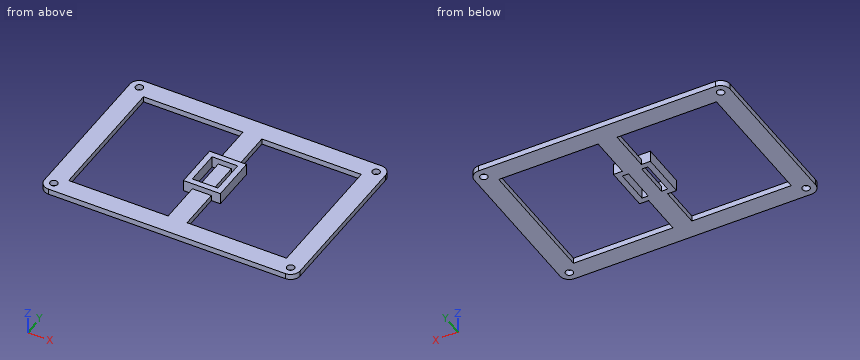
Autodesk Fusion 360 part; units mm, degrees
sketch "Boceto1" plane through (0, 0, 0) normal (0, 0, 1) x (1, 0, 0)
  line L0 (-6.75, 9.25) -> (6.75, 9.25)
  line L1 (6.75, 9.25) -> (6.75, -9.25)
  line L2 (6.75, -9.25) -> (-6.75, -9.25)
  line L3 (-6.75, -9.25) -> (-6.75, 9.25)
  line L4 (-6.75, 9.25) -> (6.75, -9.25) construction
  line L5 (6.75, 9.25) -> (-6.75, -9.25) construction
  line L6 (9.75, -12.25) -> (-9.75, -12.25)
  line L7 (-9.75, -12.25) -> (-9.75, 12.25)
  line L8 (-9.75, 12.25) -> (9.75, 12.25)
  line L9 (9.75, 12.25) -> (9.75, -12.25)
  line L10 (6.75, 0) -> (3.75, 0) construction
  line L11 (-6.75, 0) -> (-3.75, 0) construction
  line L12 (3.5, 0) -> (-3.5, 0)
  line L13 (-3.5, -9.25) -> (-3.5, 9.25)
  line L14 (3.5, -9.25) -> (3.5, 9.25)
  dimension "d1" = 13.5
  dimension "d2" = 18.5
  dimension "d3" = -3
  dimension "d4" = 3
  dimension "d5" = 3
  dimension "d6" = 7
extrude "Extruir1" add sketch "Boceto1" along normal blind 6
extrude "Extruir2" add sketch "Boceto1" along normal blind 3 contours L0 L12 L13 L14 | L2 L12 L13 L14
sketch "Boceto2" plane through (0, 0, 0) normal (0, 0, -1) x (1, 0, 0)
  line L0 (-3.5, -9.25) -> (-6.75, -9.25)
  line L1 (-6.75, -9.25) -> (-6.75, 9.25)
  line L2 (-6.75, 9.25) -> (-3.5, 9.25)
  line L3 (-3.5, 9.25) -> (-3.5, -9.25)
  line L4 (3.5, -9.25) -> (3.5, 9.25)
  line L5 (3.5, 9.25) -> (6.75, 9.25)
  line L6 (6.75, 9.25) -> (6.75, -9.25)
  line L7 (6.75, -9.25) -> (3.5, -9.25)
  line L8 (-9.75, -12.25) -> (9.75, -12.25)
  line L9 (9.75, -12.25) -> (9.75, 12.25)
  line L10 (9.75, 12.25) -> (-9.75, 12.25)
  line L11 (-9.75, 12.25) -> (-9.75, -12.25)
  line L12 (-67.5, 45) -> (67.5, 45)
  line L13 (67.5, 45) -> (67.5, -45)
  line L14 (67.5, -45) -> (-67.5, -45)
  line L15 (-67.5, -45) -> (-67.5, 45)
  line L16 (-67.5, 45) -> (67.5, -45) construction
  line L17 (67.5, 45) -> (-67.5, -45) construction
  line L18 (-67.5, 45) -> (-62.5, 45)
  line L19 (-62.5, 45) -> (-62.5, 40)
  line L20 (-67.5, -45) -> (-62.5, -45)
  line L21 (-62.5, -45) -> (-62.5, -40)
  line L22 (67.5, -45) -> (62.5, -45)
  line L23 (62.5, -45) -> (62.5, -40)
  line L24 (67.5, 45) -> (62.5, 45)
  line L25 (62.5, 45) -> (62.5, 40)
  circle A0 centre (-62.5, 40) radius 2
  circle A1 centre (-62.5, -40) radius 2
  circle A2 centre (62.5, -40) radius 2
  circle A3 centre (62.5, 40) radius 2
  line L26 (0, -12.25) -> (0, -40)
  line L27 (0, 12.25) -> (0, 40)
  line L28 (-62.5, -40) -> (-62.5, 40) construction
  line L29 (62.5, -40) -> (62.5, 40) construction
  circle A4 centre (-62.5, 40) radius 5
  circle A5 centre (62.5, 40) radius 5
  circle A6 centre (-62.5, -40) radius 5
  circle A7 centre (62.5, -40) radius 5
  line L30 (5, -40) -> (-5, -40)
  line L31 (5, 40) -> (-5, 40)
  line L32 (-5, 40) -> (-5, 12.25)
  line L33 (5, 40) -> (5, 12.25)
  line L34 (-5, -40) -> (-5, -12.25)
  line L35 (5, -40) -> (5, -12.25)
  line L36 (-62.5, -45) -> (62.5, -45)
  arc A8 (62.5, -45) -> (62.5, -35) centre (62.5, -40) ccw
  line L37 (62.5, -35) -> (-62.5, -35)
  arc A9 (-62.5, -35) -> (-62.5, -45) centre (-62.5, -40) ccw
  line L38 (-62.5, -40) -> (62.5, -40) construction
  line L39 (-62.5, 35) -> (62.5, 35)
  arc A10 (62.5, 35) -> (62.5, 45) centre (62.5, 40) ccw
  line L40 (62.5, 45) -> (-62.5, 45)
  arc A11 (-62.5, 45) -> (-62.5, 35) centre (-62.5, 40) ccw
  line L41 (-62.5, 40) -> (62.5, 40) construction
  line L42 (-57.5, -40) -> (-57.5, 40)
  arc A12 (-57.5, 40) -> (-67.5, 40) centre (-62.5, 40) ccw
  line L43 (-67.5, 40) -> (-67.5, -40)
  arc A13 (-67.5, -40) -> (-57.5, -40) centre (-62.5, -40) ccw
  line L44 (-62.5, -40) -> (-62.5, 40) construction
  line L45 (67.5, -40) -> (67.5, 40)
  arc A14 (67.5, 40) -> (57.5, 40) centre (62.5, 40) ccw
  line L46 (57.5, 40) -> (57.5, -40)
  arc A15 (57.5, -40) -> (67.5, -40) centre (62.5, -40) ccw
  line L47 (62.5, -40) -> (62.5, 40) construction
  dimension "d11" = 135
  dimension "d12" = 90
  dimension "d13" = 5
  dimension "d14" = 5
  dimension "d15" = 5
  dimension "d16" = 5
  dimension "d17" = 5
  dimension "d18" = 5
  dimension "d19" = 5
  dimension "d20" = 5
  dimension "d21" = 4
  dimension "d22" = 4
  dimension "d23" = 4
  dimension "d24" = 4
  dimension "d25" = 10
  dimension "d26" = 10
  dimension "d27" = 10
  dimension "d28" = 10
  dimension "d29" = 10
  dimension "d30" = 10
  dimension "d31" = 10
  dimension "d32" = 10
extrude "Extruir3" add sketch "Boceto2" against normal blind 3 contours L8 L26 L34 L37 | L8 L26 L35 L37 | L26 L30 L34 L37 | L14 A6 A7 L30 L34 L35 L36 L37 L42 A13 L46 A15 | L10 L27 L32 L39 | L26 L30 L35 L37 | A6 L37 L42 | L15 A4 A6 L37 A9 L39 A11 L42 L43 | L10 L27 L33 L39 | L12 A4 A5 L31 L32 L33 L39 L40 L42 A12 A14 L46 | L27 L31 L32 L39 | A6 A9 A13 | A4 L39 L42 | L27 L31 L33 L39 | L13 A5 A7 A8 L37 L39 A10 L45 L46 | A7 L37 L46 | A4 A11 A12 | A7 A8 A15 | A5 L39 L46 | A5 A10 A14
Model file for the job. Use its own axes, mm. Give positions to 0.01 mm unless a question says otherwise; leave off trailing zeros. Loops run counter-clockwise (first coordinate to the right, second up) from the corner with the lowest first, then second, coordinate; pieces in that order, holes last. Notation, with made-up numbers: M -21.5,40.25 L 1.5,40.25 A19 cw 1.5,50.25 Z; hole C -27,-22.5 d6. An arc over 180 degrees is marked long. Use one line per item in the form item = value.
Item 1: Slice it at C-C on y = -7.5. List the corners of the cut face in (x, z).
Filled in:
outline = M -67.5,0 L -57.5,0 L -57.5,3 L -67.5,3 Z; M -9.75,0 L -6.75,0 L -6.75,6 L -9.75,6 Z; M -3.5,0 L 3.5,0 L 3.5,3 L -3.5,3 Z; M 6.75,0 L 9.75,0 L 9.75,6 L 6.75,6 Z; M 57.5,0 L 67.5,0 L 67.5,3 L 57.5,3 Z
Item 2: Drill centre lines: L1, parallel to Y at x = 62.5, z = 2.15; L2, parallel to X at y = 33, z = 2.7; L3, parallel to X at y = 4.5, z = 2.4. Where is each one in solid material? Low to high.
Filled in:
L1 = -45 to -42, -38 to 38, 42 to 45
L2 = -67.5 to -57.5, -5 to 5, 57.5 to 67.5
L3 = -67.5 to -57.5, -9.75 to -6.75, -3.5 to 3.5, 6.75 to 9.75, 57.5 to 67.5
Item 3: Flat gauge pins, fed straight in: pin 1 Ø4.5 at (x, y) = (62.5, -40) entering from +Z; pin 2 Ø1.5 at (y, z) = (2, 5) entering from -X. Where does each tip first touch, or does it go through?
Filled in:
pin_1 = 3
pin_2 = -9.75
Item 4: Slice it at D-D on y = -28. List the corners of the cut face in (x, z), and give its area (3 significant figures).
Filled in:
outline = M -67.5,0 L -57.5,0 L -57.5,3 L -67.5,3 Z; M -5,0 L 5,0 L 5,3 L -5,3 Z; M 57.5,0 L 67.5,0 L 67.5,3 L 57.5,3 Z
area = 90.0 mm^2
Item 5: Slice it at B-B on z = 4.4. List the corners of the cut face in (x, y).
Filled in:
outline = M -9.75,-12.25 L 9.75,-12.25 L 9.75,12.25 L -9.75,12.25 Z; hole M -6.75,-9.25 L 6.75,-9.25 L 6.75,9.25 L -6.75,9.25 Z
Item 6: Slice it at A-A on x = 14. List the corners of the cut face in (y, z).
Filled in:
outline = M -45,0 L -35,0 L -35,3 L -45,3 Z; M 35,0 L 45,0 L 45,3 L 35,3 Z
